from build123d import *

# Parameters (mm, degrees)
MODEL_R             = 1.575
BOSS_EXTRUDE1_DEPTH = 3
FILLET1_R           = 1


with BuildPart() as part:
    # Model → Boss-Extrude1 (new body)
    with BuildSketch(Plane.XY):
        Polygon((271.203498451, 292.223209107), (291.05122826, 218.15247975), (265.115556398, 211.204247731), (260.186189629, 229.604099473), (241.30271159, 224.544411578), (243.767491017, 215.34412721), (224.664804007, 210.226469096), (223.432328054, 214.825649934), (205.733277658, 210.084029615), (206.966112962, 205.483507804), (188.744476932, 200.600523414), (190.038361872, 195.770837942), (190.009613349, 178.903688177), (183.116533861, 159.968814913), (162.674398087, 167.40803076), (131.428930231, 167.95289908), (110.986427135, 160.514692668), (104.096364698, 179.45072575), (105.814746135, 195.273012707), (107.149713912, 200.256048118), (89.106877808, 205.089769496), (90.339405557, 209.690426923), (72.639899407, 214.432169339), (71.407895987, 209.833469074), (52.305208977, 214.951127188), (54.770081908, 224.151554257), (35.886712889, 229.210569975), (30.957132238, 210.811459981), (5.0216469, 217.76022363), (25.028202346, 292.426367848), (70.198239559, 280.323200295), (72.663861356, 289.523562363), (91.063082461, 284.591613875), (92.29653696, 289.193676092), (110.695758065, 284.261727603), (109.463398178, 279.663749421), (127.862619282, 274.731800932), (126.630323598, 270.134062294), (142.522359716, 265.874644989), (142.344694619, 270.871486432), (133.979081507, 274.376202933), (135.211333861, 278.973779905), (116.812112756, 283.905728394), (118.044472643, 288.503706576), (88.054439652, 296.542595671), (86.820985153, 291.940533454), (68.42160019, 296.872525865), (65.955825932, 287.671594898), (20.785545351, 299.774827661), (-2.32684459, 213.517448416), (35.199939127, 203.463086712), (40.129543563, 221.862285479), (47.421773629, 219.90863481), (44.956891994, 210.708175253), (75.650856625, 202.485184579), (76.882860045, 207.083884844), (82.991121062, 205.447466285), (81.758593313, 200.846808858), (99.858189105, 195.997881416), (97.980730454, 178.710864183), (107.399642776, 152.824765622), (132.435827139, 161.934428279), (161.565977706, 161.426447529), (186.702312667, 152.27893851), (196.007810089, 177.840578221), (196.039346948, 196.343682115), (214.314693354, 201.241059665), (213.081966369, 205.841177268), (219.189771603, 207.477473721), (220.422247557, 202.878292884), (251.115775513, 211.101166572), (248.650938057, 220.301667543), (255.943287021, 222.255598366), (260.87259576, 203.855963236), (298.39980436, 213.909597233), (275.446186014, 299.571346393), (230.276304619, 287.470798216), (227.65276755, 297.263677376), (209.252454514, 292.334187025), (208.019481767, 296.93522173), (178.028627015, 288.898354165), (179.260689602, 284.297666211), (160.85900272, 279.367807803), (162.091473536, 274.767362889), (153.371764929, 271.263453794), (153.549484965, 266.266603363), (169.439649748, 270.524806438), (168.207287216, 275.124847165), (186.60841776, 280.054556529), (185.376246939, 284.655648642), (203.777033628, 289.586641337), (205.009898064, 284.986010813), (223.409806911, 289.915392881), (226.033325469, 280.122582817), align=None)
        with Locations((23.035554, 295.877718337)):
            Circle(MODEL_R, mode=Mode.SUBTRACT)
        with Locations((109.301822433, 156.902965293)):
            Circle(MODEL_R, mode=Mode.SUBTRACT)
        with Locations((184.800560745, 156.35733766)):
            Circle(MODEL_R, mode=Mode.SUBTRACT)
        with Locations((193.847437398, 289.84318413)):
            Circle(MODEL_R, mode=Mode.SUBTRACT)
        with Locations((102.225689846, 289.449650012)):
            Circle(MODEL_R, mode=Mode.SUBTRACT)
        with Locations((273.19609114, 295.674286852)):
            Circle(MODEL_R, mode=Mode.SUBTRACT)
        with Locations((1.570241786, 215.767496811)):
            Circle(MODEL_R, mode=Mode.SUBTRACT)
        with Locations((294.502731407, 216.159668876)):
            Circle(MODEL_R, mode=Mode.SUBTRACT)
        with Locations((80.760413887, 209.339268578)):
            Circle(MODEL_R, mode=Mode.SUBTRACT)
        with Locations((215.312231294, 209.732861073)):
            Circle(MODEL_R, mode=Mode.SUBTRACT)
    extrude(amount=-BOSS_EXTRUDE1_DEPTH)

    # Fillet1
    fillet1_edges = [part.edges().sort_by_distance(p)[0] for p in [
        (160.85900272, 279.367807803, -1.5),
        (178.028627015, 288.898354165, -1.5),
        (208.019481767, 296.93522173, -1.5),
        (227.65276755, 297.263677376, -1.5),
        (275.446186014, 299.571346393, -1.5),
        (298.39980436, 213.909597233, -1.5),
        (260.87259576, 203.855963236, -1.5),
        (251.115775513, 211.101166572, -1.5),
        (220.422247557, 202.878292884, -1.5),
        (214.314693354, 201.241059665, -1.5),
        (186.702312667, 152.27893851, -1.5),
        (107.399642776, 152.824765622, -1.5),
        (81.758593313, 200.846808858, -1.5),
        (75.650856625, 202.485184579, -1.5),
        (44.956891994, 210.708175253, -1.5),
        (35.199939127, 203.463086712, -1.5),
        (-2.32684459, 213.517448416, -1.5),
        (20.785545351, 299.774827661, -1.5),
        (65.955825932, 287.671594898, -1.5),
        (68.42160019, 296.872525865, -1.5),
        (86.820985153, 291.940533454, -1.5),
        (88.054439652, 296.542595671, -1.5),
        (118.044472643, 288.503706576, -1.5),
        (135.211333861, 278.973779905, -1.5),
    ]]
    fillet(fillet1_edges, radius=FILLET1_R)


solid = part.part
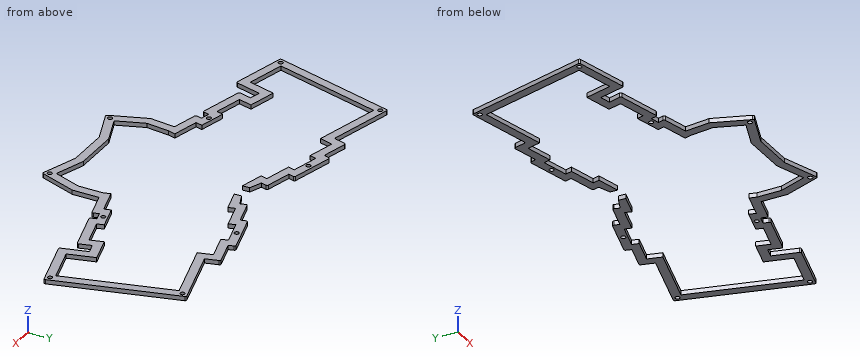
CAD build for the part. Positions are in the model's coordinates, mm. Round coordinates to 2 decimals unless told otherwise and drop trailing zeros. Write each loop counter-clockwise with the first axis right and the second up, starting at its lowest first coordinate (ties: lowest second). Pieces come first, ordered by that corner, then holes.
(1) Drop a flat-ended pin along its axis: P1, Ø1, axis at y = 190, z = -1.5, coming from the -X side. Give the stop position or say it passes through.
(2) Probe line 1 along Y through (x, z) = (79.5, -1.7); line 2 along X through (y, z) = (187, -0.3); line 3 along Y through (x, z) = (217, -1.9). List the from-to ranges inside material, lowest first.
(3) Slice it at A-A, the plane y = 261. Write the cut outline in (x, z).
(4) Slice it at B-B, the plane z = -1.5. Count the separate pieces of the cut face and the enclosed holes in it, and give its area (3 significant figures).
From the geometry:
1. P1: stops at x = 99.15
2. line 1: y = 206.38 to 208.39, 210.28 to 212.59, 287.69 to 293.9
2. line 2: x = 98.88 to 104.92, 190.02 to 196.02
2. line 3: y = 206.89 to 213.1, 288.2 to 294.41
3. outline: (10.4, -3) - (16.61, -3) - (16.61, 0) - (10.4, 0) - close; (279.57, -3) - (285.78, -3) - (285.78, 0) - (279.57, 0) - close
4. separate pieces: 1
4. enclosed holes: 10
4. area: 5,350 mm2
